Geometry: final body of the model. Coordinates: model frame, mm. A direction names the side the tool comes from. Round coordinates to 2 decimals unless told otherwise and drop trailing zeros. Loops run counter-clockwise (first coordinate to the right, second up) from the corner with the lowest first, then second, coordinate; pieces in that order, holes last. Notation, with made-up numbers: (20.5, 69.5) - (29.5, 69.5) arc R29 cw to (29.5, 103.5) - close; hole circle Ø7 at (20, -35.5). An arc over 180 degrees is marked (long way). Return JSON: item names as keys, results as strings. Group by question number.
1. First-contact query: pin 1 Ø2.5 at (y, z) = (8.5, 3.5) entering from -X; pin 2 Ø1 at (x, y) = (6, 13) entering from +Z; pin 3 Ø1.5 at (x, z) = (8.5, 13.5) entering from +Y; pin 4 Ø1.5 at (y, z) = (7, 13) entering from -X. Flat tips, straight axial feed; report the tip coordinate or a pass-through.
2. Draft query along X for faces 4 (the face through (5, 7, 12)), 5 (the face through (7, 10, 12)), 6 (the face through (10, 8, 12)), 7 (the face through (10.175, 8, 3)). Return one class per face: +X half, -X half, draft (parallel to the pull), parting line (faces both ways), or undercut.
3. Section D-D on z = 14.25. Return loops of the section in (x, y), and give its area (3 significant figures).
4. Section A-A on y = 7.5. Return loops of the section in (x, z) (3 decimals), and give its area (3 significant figures).
5. Material intervals for probe 1 along X at (y, z) = (8.75, 2.5) (3 decimals); probe 2 along Y at (x, z) = (7.25, 11.5), sorted ascending.
6. Set-up query: faces 1 (the face through (7, 10.175, 3)), 2 (the face through (4, 8, 0)), 3 (the face through (8, 5, 12)). Return all of +Z, -Z, +X, -X, +Y, -Y with unobstructed straight access to the full face (end or side cutting, diameter ignored); none if empty.
7. Section B-B on z = 3. Return loops of the section in (x, y) (3 decimals).
Autodesk Fusion 360 part; units mm, degrees
sketch "Sketch2" plane through (0, 0, 0) normal (0, 0, 1) x (1, 0, 0)
  line L0 (0, 0) -> (15, 0)
  line L1 (15, 0) -> (15, 15)
  line L2 (15, 15) -> (0, 15)
  line L3 (0, 15) -> (0, 0)
  line L4 (5, 10) -> (10, 10)
  line L5 (10, 10) -> (10, 5)
  line L6 (10, 5) -> (5, 5)
  line L7 (5, 5) -> (5, 10)
  line L8 (4.825, 10.175) -> (10.175, 10.175)
  line L9 (10.175, 10.175) -> (10.175, 4.825)
  line L10 (10.175, 4.825) -> (4.825, 4.825)
  line L11 (4.825, 4.825) -> (4.825, 10.175)
  dimension "d5" = -0.175
extrude "Extrude1" add sketch "Sketch2" along normal blind 10 contours L0 L1 L2 L3 | L8 L9 L10 L11
extrude "Extrude2" add sketch "Sketch2" along normal blind 15 contours L4 L5 L6 L7
extrude "Extrude3" cut sketch "Sketch2" along normal blind 6.175 contours L4 L5 L6 L7 | L8 L9 L10 L11
extrude "Extrude4" add 1 faces at (8.3917, 8.3917, 6.175) along direction (0, 0, -1) blind 1
Taken from the geometry:
{
 "1": {"pin 1": "x = 0", "pin 2": "z = 10", "pin 3": "y = 10", "pin 4": "x = 5"},
 "2": {"face 4": "-X half", "face 5": "draft", "face 6": "+X half", "face 7": "undercut"},
 "3": {"outline": "(5, 5) - (10, 5) - (10, 10) - (5, 10) - close", "area": "25.0 mm2"},
 "4": {"outline": "(0, 0) - (4.825, 0) - (4.825, 5.175) - (10.175, 5.175) - (10.175, 0) - (15, 0) - (15, 10) - (10, 10) - (10, 15) - (5, 15) - (5, 10) - (0, 10) - close", "area": "147 mm2"},
 "5": {"probe 1": "0 to 4.825, 10.175 to 15", "probe 2": "5 to 10"},
 "6": {"face 1": "-Z", "face 2": "-Z, +X, -X, +Y, -Y", "face 3": "+Z, +X, -X, -Y"},
 "7": {"outline": "(0, 0) - (15, 0) - (15, 15) - (0, 15) - close; hole (4.825, 4.825) - (10.175, 4.825) - (10.175, 10.175) - (4.825, 10.175) - close"}
}
